```python
from build123d import *

# Parameters (mm, degrees)
PAD_DEPTH    = 25
POCKET_DEPTH = 5


with BuildPart() as part:
    # Sketch → Pad (new body)
    with BuildSketch(Plane.XY):
        with BuildLine():
            Line((0, 0), (9.47649, 0))
            ThreePointArc((9.47649, 0), (11.59781, 0.87868), (12.47649, 3))
            Line((12.47649, 3), (12.47649, 53))
            ThreePointArc((12.47649, 53), (11.59781, 55.12132), (9.47649, 56))
            Line((9.47649, 21), (9.47649, 56))
            Line((8.47649, 21), (9.47649, 21))
            Line((8.47649, 21), (8.47649, 8))
            Line((8.47649, 8), (9.47649, 8))
            Line((9.47649, 8), (9.47649, 3))
            Line((9.47649, 3), (-9.52351, 3))
            Line((-9.52351, 3), (-9.52351, 33))
            ThreePointArc((-9.52351, 33), (-11.64483, 32.12132), (-12.52351, 30))
            Line((-12.52351, 30), (-12.52351, 13))
            Line((-12.52351, 13), (-62.52351, 13))
            Line((-62.52351, 13), (-62.52351, 10))
            Line((-62.52351, 10), (-12.52351, 10))
            Line((-12.52351, 10), (-12.52351, 3))
            ThreePointArc((-12.52351, 3), (-11.64483, 0.87868), (-9.52351, 0))
            Line((-9.52351, 0), (0, 0))
        make_face()
    extrude(amount=PAD_DEPTH)

    # Sketch001 (on Face10 of Pad) → Pocket (cut)
    with BuildSketch(Plane.XZ.offset(-10)):
        with BuildLine():
            ThreePointArc((-50, 25.000353), (-62.500176, 12.500176), (-50, 0))
            Line((-50, -4.568982), (-50, 0))
            Line((-68, -4.568982), (-50, -4.568982))
            Line((-68, 31), (-68, -4.568982))
            Line((-50, 31), (-68, 31))
            Line((-50, 25.000353), (-50, 31))
        make_face()
    extrude(amount=-POCKET_DEPTH, mode=Mode.SUBTRACT)


solid = part.part
```
CAD build for the part. Positions are in the model's coordinates, mm. A direction names the side the tool comes from. Round coordinates to 2 decimals unless told otherwise and drop trailing zeros. Write each loop counter-clockwise with the first axis right and the second up, starting at its lowest first coordinate (ties: lowest second). Pieces come first, ordered by that corner, then holes.
Item 1: Band-saw the part on D-D on x = -47. Write the cut outline in (y, z).
Filled in:
outline: (10, 0) - (13, 0) - (13, 25) - (10, 25) - close
Item 2: Band-saw the part on A-A on y = 18. Write the cut outline in (x, z).
Filled in:
outline: (-12.52, 0) - (-9.52, 0) - (-9.52, 25) - (-12.52, 25) - close; (8.48, 0) - (12.48, 0) - (12.48, 25) - (8.48, 25) - close
Item 3: Drill centre lines: L1, parallel to X at y = 15.5, z = 14.25; L2, parallel to X at y = 22, z = 7; L3, parallel to Y at x = -21, z = 6.75. Where is each one in solid material? Low to high.
Filled in:
L1: x = -12.52 to -9.52, 8.48 to 12.48
L2: x = -12.52 to -9.52, 9.48 to 12.48
L3: y = 10 to 13
Item 4: Mould opens along X. For faces 6 (the flat face through (-38, 10, 12)), 7 (the cylindrical face through (11.574, 0.855, 12.325)), 8 (the flat face through (0, 3, 12)) say: released by +X, released by -X, zero draft, split by the parting line, or undercut.
Filled in:
face 6: zero draft
face 7: released by +X
face 8: undercut
Item 5: Band-saw the part on C-C on y = 38.5. Write the cut outline in (x, z), then the cut area to 3 significant figures.
Filled in:
outline: (9.48, 0) - (12.48, 0) - (12.48, 25) - (9.48, 25) - close
area: 75.0 mm2
Item 6: Tool access for faces 1 (the flat face through (12.476, 28, 12)), 2 (the flat face through (9.476, 38, 12)), 3 (the flat face through (9.476, 6, 12)), 4 (the flat face through (-37, 13, 12)), 5 (the flat face through (-12.524, 7, 12)): list every direction of +Z, -Z, +X, -X, +Y, -Y with a clear straight run to the whole face (end or side of a thin tool).
Filled in:
face 1: +Z, -Z, +X, +Y, -Y
face 2: +Z, -Z, +Y
face 3: +Z, -Z
face 4: +Z, -Z, -X, +Y
face 5: +Z, -Z, -X, -Y
Item 7: Drop flat-ended pins along their axis: pin 1 Ø12 at (x, z) = (-51.5, 5) entering from -Y; pin 2 Ø5.5 at (y, z) = (6.5, 10) entering from -X; pin 3 Ø7.5 at (x, z) = (-29.5, 18.5) entering from +Y. Give the stop position or say it passes through.
Filled in:
pin 1: stops at y = 10
pin 2: stops at x = -12.52
pin 3: stops at y = 13
Item 8: Band-saw the part on B-B on z = 9.75. Write the cut outline in (x, y), then the cut area to 3 significant figures.
Filled in:
outline: (-62.19, 10) - (-12.52, 10) - (-12.52, 3) arc R3 ccw to (-9.52, 0) - (9.48, 0) arc R3 ccw to (12.48, 3) - (12.48, 53) arc R3 ccw to (9.48, 56) - (9.48, 21) - (8.48, 21) - (8.48, 8) - (9.48, 8) - (9.48, 3) - (-9.52, 3) - (-9.52, 33) arc R3 ccw to (-12.52, 30) - (-12.52, 13) - (-62.19, 13) - close
area: 478 mm2
